Verification items for this drawing (mm, ordinates from the low corner). A direction names the side the tool comes from. Round coordinates to 2 decimals unless told otherwise and drop trailing zeros. Write each loop counter-clockwise with the first axis right and the second up, starting at its lowest first coordinate (ties: lowest second). Pieces come first, ordered by that corner, then holes. Notation, with made-up numbers: (84, -4.5) -> (98, -4.5) arc R35 cw to (98, 30.5) -> close; hole circle Ø7 at (52, 72.5). An arc over 180 degrees is marked (long way). One line per item, written item: value.
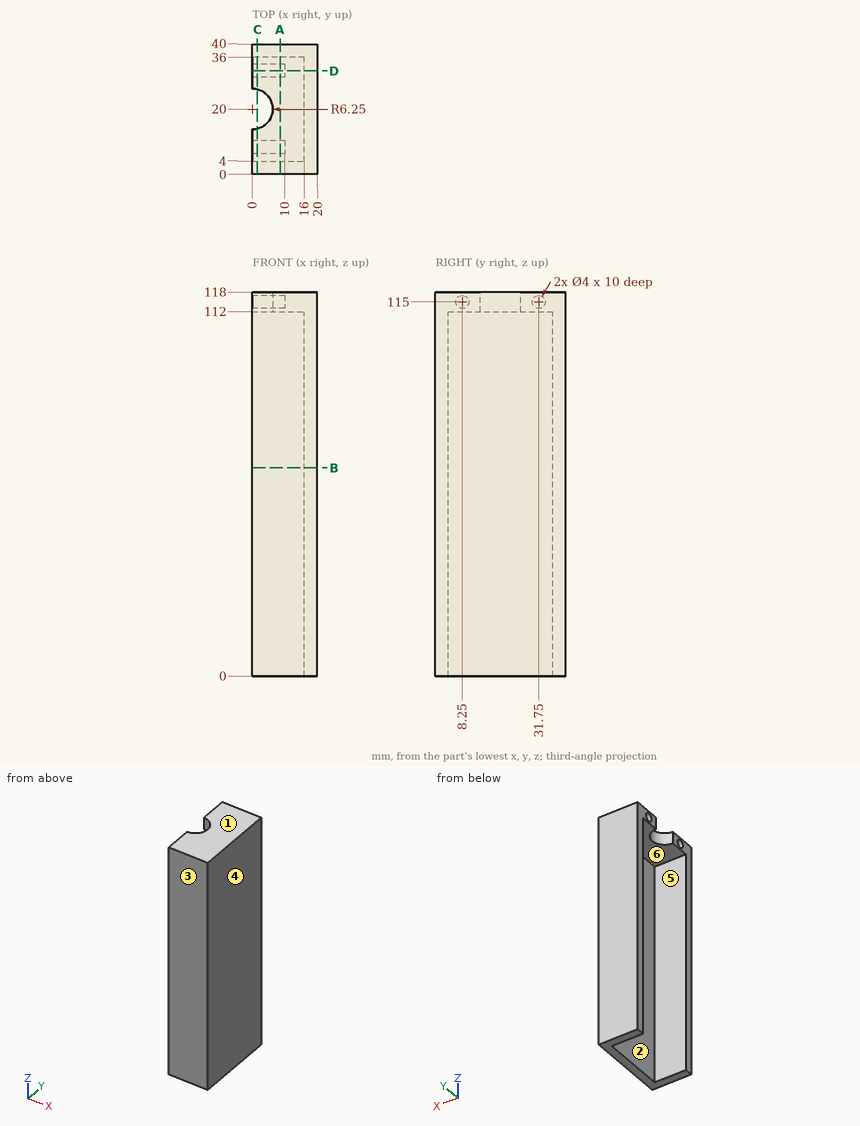
Item 1: Material ranges on line 1 along Y through (x, z) = (6.5, 115); line 2 along Y through (x, z) = (6.25, 50); line 3 along Y through (x, z) = (4.75, 115), recorded low to high.
Result set:
line 1: 0 to 6.25, 10.25 to 29.75, 33.75 to 40
line 2: 0 to 4, 36 to 40
line 3: 0 to 6.25, 10.25 to 15.94, 24.06 to 29.75, 33.75 to 40
Item 2: Sectioned sample at C-C (x = 1.5). Enter the section's corners in (y, z), then the cut area to 3 significant figures.
Result set:
outline: (0, 0) -> (4, 0) -> (4, 112) -> (13.93, 112) -> (13.93, 118) -> (0, 118) -> close; (26.07, 112) -> (36, 112) -> (36, 0) -> (40, 0) -> (40, 118) -> (26.07, 118) -> close; hole circle Ø4 at (8.25, 115); hole circle Ø4 at (31.75, 115)
area: 1,040 mm^2
Item 3: Sectioned sample at A-A (x = 8.5). Enter the section's corners in (y, z).
Result set:
outline: (0, 0) -> (4, 0) -> (4, 112) -> (36, 112) -> (36, 0) -> (40, 0) -> (40, 118) -> (0, 118) -> close; hole circle Ø4 at (8.25, 115); hole circle Ø4 at (31.75, 115)
Item 4: Sectioned sample at D-D (y = 31.75). Enter the section's corners in (x, z), then the cut area to 3 significant figures.
Result set:
outline: (0, 112) -> (16, 112) -> (16, 0) -> (20, 0) -> (20, 118) -> (0, 118) -> (0, 117) -> (10, 117) -> (10, 113) -> (0, 113) -> close
area: 528 mm^2
Item 5: Release check for a two-part mould opening along Y. For the marked faces 3, 4, 5 and 6 record: pulls with the +Y half, pulls with the -Y half, needs draft (parallel to the pull), parting line crosses it, or undercut.
Result set:
face 3: pulls with the -Y half
face 4: needs draft
face 5: undercut
face 6: undercut
Item 6: Tool access check on the marked faces 1 and 2. Record the directions out of +Z, -Z, +X, -X, +Y, -Y that give a thin tool (end or side, any length) a straight path to the whole face; none if there is none.
Result set:
face 1: +Z, +X, -X, +Y, -Y
face 2: -Z, -X
Item 7: Depth check by flat-ended pin: pin 1 (5 mm diameter, centred on y = 30, z = 65, fed in from -X); pin 2 (5 mm diameter, centred on x = 8, y = 13, fed in from -Z). Enter the tip coordinate at first touch or a pass-through.
Result set:
pin 1: x = 16
pin 2: z = 112
Item 8: Sectioned sample at B-B (z = 64). Enter the section's corners in (x, y).
Result set:
outline: (0, 0) -> (20, 0) -> (20, 40) -> (0, 40) -> (0, 36) -> (16, 36) -> (16, 4) -> (0, 4) -> close
